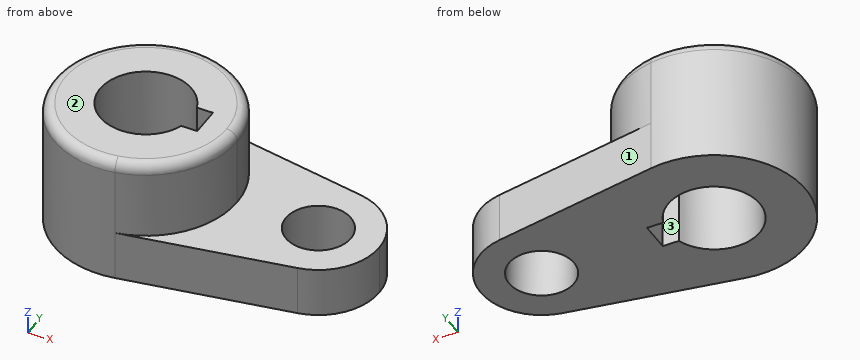
from build123d import *

# Parameters (mm, degrees)
F1_DEPTH = 40.2336
F0_R     = 10.16
F2_DEPTH = 15.7734
F3_R     = 3.302


with BuildPart() as f1:
    # F0 (on Top) → F1 (new body)
    with BuildSketch(Plane.XY):
        with BuildLine():
            ThreePointArc((5.042647, -28.126541), (21.916025, -18.336262), (28.575, 0))
            ThreePointArc((28.575, 0), (21.916025, 18.336262), (5.042647, 28.126541))
            ThreePointArc((5.042647, 28.126541), (-28.575, 0), (5.042647, -28.126541))
        make_face()
        with BuildLine():
            ThreePointArc((13.497268, -4.685767), (-14.2875, 0), (13.497268, 4.685767))
            Line((13.497268, 4.685767), (18.5293, 4.685767))
            Line((18.5293, 4.685767), (18.5293, -4.685767))
            Line((18.5293, -4.685767), (13.497268, -4.685767))
        make_face(mode=Mode.SUBTRACT)
    extrude(amount=F1_DEPTH)

    # F0 (on Top) → F2 (join)
    with BuildSketch(Plane.XY):
        with BuildLine():
            ThreePointArc((5.042647, -28.126541), (21.916025, -18.336262), (28.575, 0))
            ThreePointArc((28.575, 0), (21.916025, 18.336262), (5.042647, 28.126541))
            ThreePointArc((5.042647, 28.126541), (-28.575, 0), (5.042647, -28.126541))
        make_face()
        with BuildLine():
            ThreePointArc((13.497268, -4.685767), (-14.2875, 0), (13.497268, 4.685767))
            Line((13.497268, 4.685767), (18.5293, 4.685767))
            Line((18.5293, 4.685767), (18.5293, -4.685767))
            Line((18.5293, -4.685767), (13.497268, -4.685767))
        make_face(mode=Mode.SUBTRACT)
        with BuildLine():
            ThreePointArc((5.042647, 28.126541), (21.916025, 18.336262), (28.575, 0))
            ThreePointArc((28.575, 0), (21.916025, -18.336262), (5.042647, -28.126541))
            Line((5.042647, -28.126541), (57.336765, -18.751028))
            ThreePointArc((57.336765, -18.751028), (34.925, 0), (57.336765, 18.751028))
            Line((57.336765, 18.751028), (5.042647, 28.126541))
        make_face()
        with BuildLine():
            ThreePointArc((73.025, 0), (68.585683, 12.224174), (57.336765, 18.751028))
            ThreePointArc((57.336765, 18.751028), (34.925, 0), (57.336765, -18.751028))
            ThreePointArc((57.336765, -18.751028), (68.585683, -12.224174), (73.025, 0))
        make_face()
        with Locations((53.975, 0)):
            Circle(F0_R, mode=Mode.SUBTRACT)
    extrude(amount=F2_DEPTH)

    # F3
    f3_edges = [f1.edges().sort_by_distance(p)[0] for p in [
        (-5.042647, 28.126541, 40.2336),
    ]]
    fillet(f3_edges, radius=F3_R)


solid = f1.part
Input: part model. Units: mm. Frame: model coordinates. Face numbers are marked on the shaded views. Coordinates: 2 decimals unless noted, no trailing zeros.
(1) Section B-B on y = -9. Count the separate pieces of the cut face and the enclosed holes in it, then the cut area to 3 significant figures.
(2) Material intervals for probe 1 along Y at (x, z) = (0, 14) (1 decimal); probe 2 along X at (y, z) = (-5, 28.5); probe 3 along X at (y, z) = (11, 13.5), sorted ascending.
(3) First-contact query: pin 1 Ø7.5 at (y, z) = (1.5, 17.5) entering from -X (3 decimals); pin 2 Ø5 at (y, z) = (8.5, 21.5) entering from +X; pin 3 Ø5 at (x, z) = (6.5, 18) entering from -Y. Flat tips, straight axial feed; report the tip coordinate or a pass-through.
(4) Pull-direction query (Y, two-part tool) for the marked faces 1, 2 and 3; classes: released by +Y, released by -Y, zero draft, split by the parting line, or undercut.
Data:
1. separate pieces: 3
1. enclosed holes: 0
1. area: 1,820 mm2
2. probe 1: y = -28.6 to -14.3, 14.3 to 28.6
2. probe 2: x = -28.13 to -13.38, 13.38 to 28.13
2. probe 3: x = -26.37 to -9.12, 9.12 to 69.53
3. pin 1: stops at x = -28.575
3. pin 2: stops at x = 27.94
3. pin 3: stops at y = -28.29
4. face 1: released by +Y
4. face 2: zero draft
4. face 3: undercut
